from build123d import *

# Parameters (mm, degrees)
SKETCH1_W                                       = 60
SKETCH1_H                                       = 120
BOSS_EXTRUDE1_DEPTH                             = 6.54
SKETCH10_W                                      = 6.54
SKETCH10_H                                      = 45
BOSS_EXTRUDE5_DEPTH                             = 17
SKETCH17_W                                      = 60
SKETCH17_H                                      = 40
BOSS_EXTRUDE6_DEPTH                             = 29
CUT_EXTRUDE1_REACH                              = 42
CUT_EXTRUDE2_REACH                              = 54.54
SKETCH21_W                                      = 37.9445377
SKETCH21_H                                      = 40
SKETCH23_W                                      = 2
SKETCH23_H                                      = 36
CUT_EXTRUDE3_DEPTH                              = 9
SKETCH24_W                                      = 2
SKETCH24_H                                      = 36
CUT_EXTRUDE4_DEPTH                              = 9
CSK_FOR_M3_FLAT_HEAD_MACHINE_SCREW4_D           = 4.93
CSK_FOR_M3_FLAT_HEAD_MACHINE_SCREW4_DEPTH       = 6.54
CSK_FOR_M3_FLAT_HEAD_MACHINE_SCREW4_CSINK_D     = 12
CSK_FOR_M3_FLAT_HEAD_MACHINE_SCREW4_CSINK_ANGLE = 90
CSK_FOR_M3_FLAT_HEAD_MACHINE_SCREW5_D           = 4.93
CSK_FOR_M3_FLAT_HEAD_MACHINE_SCREW5_DEPTH       = 6.54
CSK_FOR_M3_FLAT_HEAD_MACHINE_SCREW5_CSINK_D     = 12
CSK_FOR_M3_FLAT_HEAD_MACHINE_SCREW5_CSINK_ANGLE = 90
BOSS_EXTRUDE8_DEPTH                             = 29
SKETCH36_W                                      = 60
SKETCH36_H                                      = 1.8
BOSS_EXTRUDE9_DEPTH                             = 6.5
FILLET1_R                                       = 3
FILLET2_R                                       = 2


with BuildPart() as part:
    # Sketch1 → Boss-Extrude1 (new body)
    with BuildSketch(Plane.XY):
        Rectangle(SKETCH1_W, SKETCH1_H)
    extrude(amount=BOSS_EXTRUDE1_DEPTH)

    # Sketch10 → Boss-Extrude5 (add)
    with BuildSketch(Plane(origin=(0, 0, 0), x_dir=(-1, 0, 0), z_dir=(0, 0, -1))):
        with Locations((23.27, -2.5)):
            Rectangle(SKETCH10_W, SKETCH10_H)
        with Locations((-23.27, -2.5)):
            Rectangle(SKETCH10_W, SKETCH10_H)
    extrude(amount=BOSS_EXTRUDE5_DEPTH)

    # Sketch17 → Boss-Extrude6 (add)
    with BuildSketch(Plane.XY.offset(6.54)):
        with Locations((0, -40)):
            Rectangle(SKETCH17_W, SKETCH17_H)
    extrude(amount=BOSS_EXTRUDE6_DEPTH)

    # Sketch18 → Cut-Extrude1 (cut, up to next)
    with BuildSketch(Plane(origin=(0, -20, 0), x_dir=(1, 0, 0), z_dir=(0, 1, 0)), mode=Mode.PRIVATE) as cut_extrude1_sk1:
        with BuildLine():
            Line((5.334966353, -8.526396136), (21.291300905, -12.825812438))
            add(Edge.make_bspline(
                [(5.334966353, -8.526396136), (-17.854714365, -9.780670981), (-12.49786254, -23.648890313), (-7.141010715, -37.517109645), (13.926544327, -30.768916863), (34.994099369, -24.020724082), (21.291300905, -12.825812438)],
                knots=[1.570796327, 1.570796327, 1.570796327, 3.340987112, 3.340987112, 5.111177898, 5.111177898, 6.881368684, 6.881368684, 6.881368684], degree=2, weights=[1, 0.633215673, 1, 0.633215673, 1, 0.633215673, 1]))
        make_face()
    cut_extrude1_tool1 = extrude(cut_extrude1_sk1.sketch, amount=-CUT_EXTRUDE1_REACH, mode=Mode.PRIVATE) & part.part
    add(cut_extrude1_tool1.solids().sort_by_distance((5.792514, -20, 20.554542))[0], mode=Mode.SUBTRACT)

    # Sketch21 → Cut-Extrude2 (cut, up to next)
    with BuildSketch(Plane.XY.offset(35.54), mode=Mode.PRIVATE) as cut_extrude2_sk1:
        with Locations((5.97226885, -40)):
            Rectangle(SKETCH21_W, SKETCH21_H)
    cut_extrude2_tool1 = extrude(cut_extrude2_sk1.sketch, amount=-CUT_EXTRUDE2_REACH, mode=Mode.PRIVATE) & part.part
    add(cut_extrude2_tool1.solids().sort_by_distance((5.972269, -40, 35.54))[0], mode=Mode.SUBTRACT)

    # Sketch23 → Cut-Extrude3 (cut)
    with BuildSketch(Plane(origin=(-13, 0, 0), x_dir=(0, 0, -1), z_dir=(1, 0, 0))):
        with Locations((-33.04, -40)):
            Rectangle(SKETCH23_W, SKETCH23_H)
    extrude(amount=-CUT_EXTRUDE3_DEPTH, mode=Mode.SUBTRACT)

    # Sketch24 → Cut-Extrude4 (cut)
    with BuildSketch(Plane.ZY.offset(-24.9445377)):
        with Locations((33.04, -40)):
            Rectangle(SKETCH24_W, SKETCH24_H)
    extrude(amount=-CUT_EXTRUDE4_DEPTH, mode=Mode.SUBTRACT)

    # CSK for M3 Flat Head Machine Screw4
    with Locations(Plane(origin=(26.54, -12.5, -10), x_dir=(0, 1, 0), z_dir=(1, 0, 0))):
        with Locations((0, 0), (20, 0)):
            CounterSinkHole(CSK_FOR_M3_FLAT_HEAD_MACHINE_SCREW4_D / 2, CSK_FOR_M3_FLAT_HEAD_MACHINE_SCREW4_CSINK_D / 2, depth=CSK_FOR_M3_FLAT_HEAD_MACHINE_SCREW4_DEPTH, counter_sink_angle=CSK_FOR_M3_FLAT_HEAD_MACHINE_SCREW4_CSINK_ANGLE)

    # CSK for M3 Flat Head Machine Screw5
    with Locations(Plane(origin=(-26.54, -12.5, -10), x_dir=(0, -1, 0), z_dir=(-1, 0, 0))):
        with Locations((0, 0), (-20, 0)):
            CounterSinkHole(CSK_FOR_M3_FLAT_HEAD_MACHINE_SCREW5_D / 2, CSK_FOR_M3_FLAT_HEAD_MACHINE_SCREW5_CSINK_D / 2, depth=CSK_FOR_M3_FLAT_HEAD_MACHINE_SCREW5_DEPTH, counter_sink_angle=CSK_FOR_M3_FLAT_HEAD_MACHINE_SCREW5_CSINK_ANGLE)

    # Sketch7 → Boss-Extrude8 (add)
    with BuildSketch(Plane.XY.offset(6.54)):
        with BuildLine():
            Line((-10, 25.533918981), (-18.67330273, 45.101562584))
            ThreePointArc((-18.67330273, 45.101562584), (-20, 46), (-21.305734932, 45.071360283))
            Line((-21.305734932, 45.071360283), (-30, 29.115374119))
            Line((-30, 29.115374119), (-30, 25.533918981))
            Line((-30, 25.533918981), (-10, 25.533918981))
        make_face()
    extrude(amount=BOSS_EXTRUDE8_DEPTH)

    # Sketch36 → Boss-Extrude9 (add)
    with BuildSketch(Plane.XY.offset(6.54)):
        with Locations((0, 54.4)):
            Rectangle(SKETCH36_W, SKETCH36_H)
    extrude(amount=BOSS_EXTRUDE9_DEPTH)

    # Fillet1
    fillet1_edges = [part.edges().sort_by_distance(p)[0] for p in [
        (-10, 25.533918981, 21.04),
    ]]
    fillet(fillet1_edges, radius=FILLET1_R)

    # Fillet2
    fillet2_edges = [part.edges().sort_by_distance(p)[0] for p in [
        (-30, 25.533918981, 21.04),
    ]]
    fillet(fillet2_edges, radius=FILLET2_R)


solid = part.part
Read the model definition and answer for the solid it produces. Units are mm, in the model's axes. A direction names the side the tool comes from. Coordinates: 2 decimals unless noted, no trailing zeros. Write each loop counter-clockwise with the first axis right and the second up, starting at its lowest first coordinate (ties: lowest second). Pieces come first, ordered by that corner, then holes. Notation, with made-up numbers: (-37.75, 66) -> (-17.75, 66) arc R16 ccw to (-17.75, 85) -> close; hole circle Ø4 at (45.25, 42.5). An arc over 180 degrees is marked (long way). Return JSON: item names as keys, results as strings.
(1) Each of these flat-tipped pins is pushed along its axis until it touches: P1, Ø14.5, axis at x = -1.5, z = 24.5, coming from the +Y side; P2, Ø7, axis at x = -22.5, z = -10.5, coming from the -Y side; P3, Ø8, axis at x = 10.5, y = 35.5, coming from the -Z side; P4, Ø2, axis at x = -16.5, z = 33, coming from the +Y side. Where does it stop, or does it pass through?
Answers below:
{"P1": "through", "P2": "y = -25", "P3": "z = 0", "P4": "y = 42.45"}
(2) The part is cut by section C-C on x = -16. Give the vertices of the cut face in (y, z), then the cut area to 3 significant figures.
Answers below:
{"outline": "(-60, 0) -> (60, 0) -> (60, 6.54) -> (55.3, 6.54) -> (55.3, 13.04) -> (53.5, 13.04) -> (53.5, 6.54) -> (39.07, 6.54) -> (39.07, 35.54) -> (25.53, 35.54) -> (25.53, 6.54) -> (-20, 6.54) -> (-20, 35.54) -> (-60, 35.54) -> close; hole (-58, 32.04) -> (-22, 32.04) -> (-22, 34.04) -> (-58, 34.04) -> close", "area": "2,280 mm^2"}
(3) For a pull along Z with two mould halves and no side action, classify faces 5 (the flat face through (26.54, -3, -8)), 6 (the flat face through (23, -2, -17)), 7 (the flat face through (-22, -40, 35.54)), 8 (the flat face through (-17, -40, 34.04)) as pulls with the +Z half, pulls with the -Z half, needs draft (parallel to the pull), parting line crosses it, or undercut.
Answers below:
{"face 5": "needs draft", "face 6": "pulls with the -Z half", "face 7": "pulls with the +Z half", "face 8": "undercut"}
(4) Which of the six approach directions +Z, -Z, +X, -X, +Y, -Y give full straight-line access (tool end or side, diameter ignored) to faces 1 (the flat face through (23, -25, -8)), 2 (the flat face through (-25.59, 37.21, 20.84)), 3 (the flat face through (-14, -20, 18)), 4 (the flat face through (-13, -40, 29))?
Answers below:
{"face 1": "-Z, +X, -X, -Y", "face 2": "+Z, -X", "face 3": "+Z, +X, -X", "face 4": "+Z, -Y"}
(5) Consider line 1 along Y through (x, z) = (-22.3, -10) (3 decimals); line 2 along X through (y, z) = (-30.5, 31); line 3 along Y through (x, z) = (17, 9.5). Determine where each line is inside the solid, lowest interval first. Write a range as from..to.
Answers below:
{"line 1": "-25..-14.965, -10.035..5.035, 9.965..20", "line 2": "-30..-13, 24.94..30", "line 3": "-60..-20, 53.5..55.3"}
(6) The part is cut by section D-D on y = 42.5. Give the vertices of the cut face in (x, z).
Answers below:
{"outline": "(-30, 0) -> (30, 0) -> (30, 6.54) -> (-17.52, 6.54) -> (-17.52, 35.54) -> (-22.71, 35.54) -> (-22.71, 6.54) -> (-30, 6.54) -> close"}
(7) The part is cut by section A-A on y = -12.5. Give the vertices of the cut face in (x, z) (3 decimals), then the cut area to 3 significant figures.
Answers below:
{"outline": "(-30, 0) -> (-26.54, 0) -> (-26.54, -4) -> (-23.005, -7.535) -> (-20, -7.535) -> (-20, 0) -> (20, 0) -> (20, -7.535) -> (23.005, -7.535) -> (26.54, -4) -> (26.54, 0) -> (30, 0) -> (30, 6.54) -> (-30, 6.54) -> close; (-26.54, -17) -> (-20, -17) -> (-20, -12.465) -> (-23.005, -12.465) -> (-26.54, -16) -> close; (20, -17) -> (26.54, -17) -> (26.54, -16) -> (23.005, -12.465) -> (20, -12.465) -> close", "area": "525 mm^2"}
(8) The part is cut by section B-B on z = -10. State how many separate pieces and enclosed holes the cut face has, then the cut area to 3 significant figures.
Answers below:
{"separate pieces": "6", "enclosed holes": "0", "area": "410 mm^2"}
